Could you check a few things on this model? Use its own coordinates, in mm. A direction names the side the tool comes from. Give positions to 0.01 mm unless a question says otherwise; leave off trailing zeros. Order: outer loops, then holes, each group sorted by start corner. A loop starts at its lowest first (then second) coordinate and runs counter-clockwise, first axis right, second up. Notation, with made-up numbers: (31, 68) -> (53, 68) arc R35 cw to (53, 106) -> close; hole circle Ø5 at (-27.5, 61.25). An arc over 180 degrees is marked (long way). Write each question's results on one line, items separated by ' | '.
Autodesk Inventor part; units mm, degrees
ref_plane "YZ Plane" through (0, 0, 0) normal (1, 0, 0) x (0, 1, 0)
ref_plane "XZ Plane" through (0, 0, 0) normal (0, 1, 0) x (-1, 0, 0)
ref_plane "XY Plane" through (0, 0, 0) normal (0, 0, 1) x (1, 0, 0)
sketch "Skizze1" plane through (0, 0, 0) normal (0, 0, 1) x (1, 0, 0)
  line L0 (0, 0) -> (0, 60.5) construction
  line L1 (0, 0) -> (-8, 0)
  line L2 (-8, 0) -> (-8, 5)
  line L3 (-8, 5) -> (-17.5, 5)
  line L4 (-17.5, 5) -> (-17.5, 11)
  line L5 (-17.5, 11) -> (-8, 21)
  line L6 (-8, 21) -> (-5.5, 55.3854)
  arc A0 (5.5, 55.3854) -> (-5.5, 55.3854) centre (0, 54.9855) ccw
  line L7 (5.5, 55.3854) -> (8, 21)
  line L8 (8, 21) -> (17.5, 11)
  line L9 (17.5, 11) -> (17.5, 5)
  line L10 (17.5, 5) -> (8, 5)
  line L11 (8, 5) -> (8, 0)
  line L12 (8, 0) -> (0, 0)
  dimension "d6" = 60.5
  dimension "d7" = 16
  dimension "d8" = 5
  dimension "d9" = 11
  dimension "d10" = 35
  dimension "d11" = 11
  dimension "d12" = 21
extrude "Extrusion1" add sketch "Skizze1" along normal blind 10
sketch "Skizze2" plane through (0, 0, 10) normal (0, 0, 1) x (1, 0, 0)
  line L0 (-8, 0) -> (8, 0)
  arc A0 (6, 0) -> (-6, 0) centre (0, 0) ccw
  point P0 (0, 0)
  dimension "d15" = 12
extrude "Extrusion2" cut sketch "Skizze2" against normal blind 10
sketch "Skizze3" plane through (-17.5, 5, 0) normal (0, -1, 0) x (1, 0, 0)
  line L0 (17.5, 0) -> (17.5, 10) construction
  line L1 (11.5, 10) -> (23.5, 10)
  line L2 (0, 0) -> (0, 10)
  point P0 (4.75, 5)
  point P1 (30.25, 5)
  point P2 (0, 5)
  dimension "d18" = 25.5
hole "Bohrung1" at (-12.75, 5, 5) at (12.75, 5, 5) direction (0, 1, 0) diameter 3.242 depth 9 tip angle 118
sketch "Skizze4" plane through (0, 0, 10) normal (0, 0, 1) x (1, 0, 0)
  arc A0 (5.5, 55.3854) -> (-5.5, 55.3854) centre (0, 54.9855) ccw
  point P0 (0, 0)
hole "Bohrung2" at (0, 54.9855, 10) direction (0, 0, -1) diameter 6.02 end through all
properties part number "Pleuel_oberteil" material "Stahl, galvanisiert"
Q1. Suppose I cut it at D-D on y = 22. Please give me the cut outline in (x, z), and give its area (3 significant figures).
Here are the results:
outline: (-7.93, 0) -> (7.93, 0) -> (7.93, 10) -> (-7.93, 10) -> close | area: 159 mm²
Q2. Suppose I cut it at C-C on y = 8. Please give me the cut outline in (x, z).
Here are the results:
outline: (-17.5, 0) -> (17.5, 0) -> (17.5, 10) -> (-17.5, 10) -> close; hole circle Ø3.24 at (-12.75, 5); hole circle Ø3.24 at (12.75, 5)
Q3. Suppose I cut it at B-B on x = 0. Please give me the cut outline in (y, z), and give its area (3 significant figures).
Here are the results:
outline: (6, 0) -> (51.98, 0) -> (51.98, 10) -> (6, 10) -> close; (58, 0) -> (60.5, 0) -> (60.5, 10) -> (58, 10) -> close | area: 485 mm²
Q4. I need wall thicknesses on line 1 along X through (y, z) = (7.75, 5); line 2 along X through (y, z) = (11.5, 5) (3 decimals); line 3 along Z through (x, y) = (12.75, 10.5). Which ranges of each line are inside material? Lowest first, please.
Here are the results:
line 1: x = -17.5 to -14.37, -11.13 to 11.13, 14.37 to 17.5 | line 2: x = -17.025 to -14.371, -11.129 to 11.129, 14.371 to 17.025 | line 3: z = 0 to 3.38, 6.62 to 10
Q5. Suppose I cut it at A-A on z = 2. Please give me the cut outline in (x, y), and give its area (3 significant figures).
Here are the results:
outline: (-17.5, 5) -> (-8, 5) -> (-8, 0) -> (-6, 0) arc R6 cw to (6, 0) -> (8, 0) -> (8, 5) -> (17.5, 5) -> (17.5, 11) -> (8, 21) -> (5.5, 55.39) arc R5.51 ccw to (-5.5, 55.39) -> (-8, 21) -> (-17.5, 11) -> close; hole circle Ø6.02 at (0, 54.99) | area: 968 mm²
Q6. I'm going to push flat-ended pins straight in: pin 1 Ø3.5 at (x, z) = (-12.75, 5) entering from -Y; pin 2 Ø3 at (y, z) = (43.5, 3.5) entering from +X; pin 3 Ø2.5 at (y, z) = (3, 4.5) entering from +X. Where does each tip first touch, or does it pass through?
Here are the results:
pin 1: stops at y = 5 | pin 2: stops at x = 6.47 | pin 3: stops at x = 8
Q7. Thinking about a two-plate mould opening in Y: for faces 1 (the cylindrical face through (11.143, 9.563, 5.211)), 2 (the cylindrical face through (1.153, 52.205, 4.93)), 3 (the flat face through (-12.817, 15.93, 4.93)), which applies, +Y half, -Y half, draft (parallel to the pull), parting line (faces both ways), or undercut?
Here are the results:
face 1: draft | face 2: undercut | face 3: +Y half
Q8. For faces 4 (the flat face through (12.683, 16.07, 4.93)), 5 (the cylindrical face through (-14.357, 9.563, 5.211)), 6 (the flat face through (-10.6, 5, 4.9)), 7 (the flat face through (15, 5, 5)), 8 (the flat face through (-6.768, 37.952, 4.93)), which set-ups out of +Z, -Z, +X, -X, +Y, -Y let a thin tool reach every point of the face, with its end or its side?
Here are the results:
face 4: +Z, -Z, +X, +Y | face 5: -Y | face 6: +Z, -Z, -X, -Y | face 7: +Z, -Z, +X, -Y | face 8: +Z, -Z, -X, +Y
